Model file for the job. Use its own axes, mm. Face numbers are marked on the shaded views. A direction names the side the tool comes from. Round coordinates to 2 decimals unless told otherwise and drop trailing zeros. Order: outer loops, then holes, each group sorted by start corner. A loop starts at its lowest first (then second) coordinate and runs counter-clockwise, first axis right, second up. Notation, with made-up numbers: M -28.5,41.5 L -5.5,41.5 A14 cw -5.5,54.5 Z; hole C -19,-2.75 d1. An arc over 180 degrees is marked long. Return JSON: item names as keys, results as strings. Group by question number.
Item 1: Slice it at D-D on x = 16. Write the cut outline in (y, z), then the cut area to 3 significant figures.
Item 2: Which spindle directions (+Z, -Z, +X, -X, +Y, -Y) get a long thin tool onto all of the face, cutting with end or side? Do the marked faces 1, 2 and 3. Say none if no direction does.
Item 3: Pull direction Z, two halves, no side cores. Call the marked faces 4, 5 and 6: pulls with the +Z half, pulls with the -Z half, needs draft (parallel to the pull), parting line crosses it, or undercut.
Item 4: Pin check, flat tips, straight feed: pin 1 Ø1.1 at (x, y) = (-6, 5.5) entering from -Z (3 decimals); pin 2 Ø8 at (x, z) = (-4, 20.5) entering from -Y; pin 3 Ø2 at (x, y) = (-18, 2) entering from -Z. Stop position of each tip, or through.
Item 5: Probe line 1 along Z through (x, y) = (0, 3.05); line 2 along X through (y, z) = (3.9, 0); line 3 along X through (y, z) = (3.5, 16). List the from-to ranges inside material, lowest first.
Item 6: Slice it at A-A on x = 0. Write the cut outline in (y, z), then the cut area to 4 significant figures.
Item 7: Slice it at B-B on z = 0. Write the cut outline in (x, y).
Item 8: Slice it at C-C on z = -26. Write the cut outline in (x, y).
from build123d import *

# Parameters (mm, degrees)
BASE_R                     = 30.25
EXTRUSAO_BASE_DEPTH        = 8
CORTE_BASE_R               = 28.75
EXTRUSAO_CORTE_BASE_DEPTH  = 5
USB_W                      = 142.526664036
USB_H                      = 12
CORTE_USB_DEPTH            = 6.5
CORTE_PRISMA_DEPTH         = 44.521546388
CORTE_PRISMA_DEPTH_BACK    = 44.521546388
PRISMA2_W                  = 15
PRISMA2_H                  = 15
PRISMA_W                   = 27
PRISMA_H                   = 27
CORTE_ENCAIXE_PRISMA_DEPTH = 2


with BuildPart() as part:
    # base → extrusao_base (new body)
    with BuildSketch(Plane(origin=(0, 0, 0), x_dir=(1, 0, 0), z_dir=(0, 1, 0))):
        with Locations(Location((0, 0, 0), (0, 0, 270))):
            Circle(BASE_R)
    extrude(amount=EXTRUSAO_BASE_DEPTH)

    # corte_base → extrusao_corte_base (cut)
    with BuildSketch(Plane(origin=(0, 0, 0), x_dir=(1, 0, 0), z_dir=(0, 1, 0))):
        with Locations(Location((0, 0, 0), (0, 0, 270))):
            Circle(CORTE_BASE_R)
    extrude(amount=EXTRUSAO_CORTE_BASE_DEPTH, mode=Mode.SUBTRACT)

    # usb → corte_usb (cut)
    with BuildSketch(Plane(origin=(0, 0, 0), x_dir=(1, 0, 0), z_dir=(0, 1, 0))):
        with Locations((-71.263332018, 0)):
            Rectangle(USB_W, USB_H)
    extrude(amount=CORTE_USB_DEPTH, mode=Mode.SUBTRACT)

    # prisma2 (on Top Plane) → corte_prisma (cut, two sides: drawn at the far end of the back side and taken through both)
    with BuildSketch(Plane(origin=(0, 0, 0), x_dir=(1, 0, 0), z_dir=(0, 1, 0)).offset(-CORTE_PRISMA_DEPTH_BACK)):
        with Locations((-6.438503074, 0)):
            Rectangle(PRISMA2_W, PRISMA2_H)
    extrude(amount=CORTE_PRISMA_DEPTH + CORTE_PRISMA_DEPTH_BACK, mode=Mode.SUBTRACT)

    # prisma → corte_encaixe_prisma (cut)
    with BuildSketch(Plane(origin=(0, 8, 0), x_dir=(1, 0, 0), z_dir=(0, 1, 0))):
        with Locations((-6.438503074, 0)):
            Rectangle(PRISMA_W, PRISMA_H)
    extrude(amount=-CORTE_ENCAIXE_PRISMA_DEPTH, mode=Mode.SUBTRACT)


solid = part.part
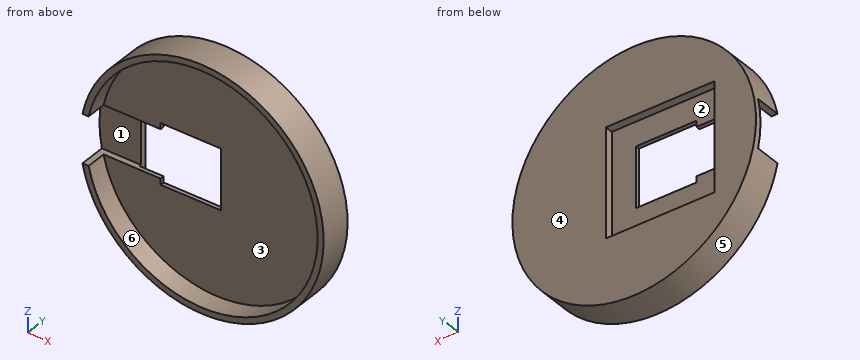
Output values:
{
 "1": {"outline": "M 0,-25.67 L 8,-25.67 L 8,25.67 L 0,25.67 L 0,23.89 L 5,23.89 L 5,-23.89 L 0,-23.89 Z", "area": "172 mm²"},
 "2": {"face 1": "-X, -Y", "face 2": "+Y", "face 3": "-Y"},
 "3": {"face 4": "needs draft", "face 5": "parting line crosses it", "face 6": "undercut"},
 "4": {"pin 1": "z = -29.755", "pin 2": "y = 5", "pin 3": "z = -25.02"},
 "5": {"line 1": "-30.25 to -28.75, 28.75 to 30.25", "line 2": "28.75 to 30.25", "line 3": "-25.67 to -23.89, 23.89 to 25.67"},
 "6": {"outline": "M 0,-30.25 L 8,-30.25 L 8,-13.5 L 6,-13.5 L 6,-7.5 L 5,-7.5 L 5,-28.75 L 0,-28.75 Z; M 0,28.75 L 5,28.75 L 5,7.5 L 6,7.5 L 6,13.5 L 8,13.5 L 8,30.25 L 0,30.25 Z", "area": "127.5 mm²"},
 "7": {"outline": "M -30.25,6.5 L -19.94,6.5 L -19.94,8 L -30.25,8 Z; M 1.06,5 L 28.75,5 L 28.75,0 L 30.25,0 L 30.25,8 L 7.06,8 L 7.06,6 L 1.06,6 Z"},
 "8": {"outline": "M -15.46,0 L -12.27,0 L -12.27,5 L 12.27,5 L 12.27,0 L 15.46,0 L 15.46,8 L -15.46,8 Z"}
}
